Geometry check sheet. Reference: drawing and pictorial views, mm from the part's lowest x, y, z. Give positions to 0.01 mm unless a question says otherwise; leave off trailing zeros. Loops run counter-clockwise (first coordinate to the right, second up) from the corner with the lowest first, then second, coordinate; pieces in that order, holes last. Notation, with made-up numbers: M 61,-3.5 L 88,-3.5 A4 ccw 88,0.5 Z; hole C 11,74.25 d8. An arc over 180 degrees is marked long. Put each result on its own line as item: value. Start each with the question number.
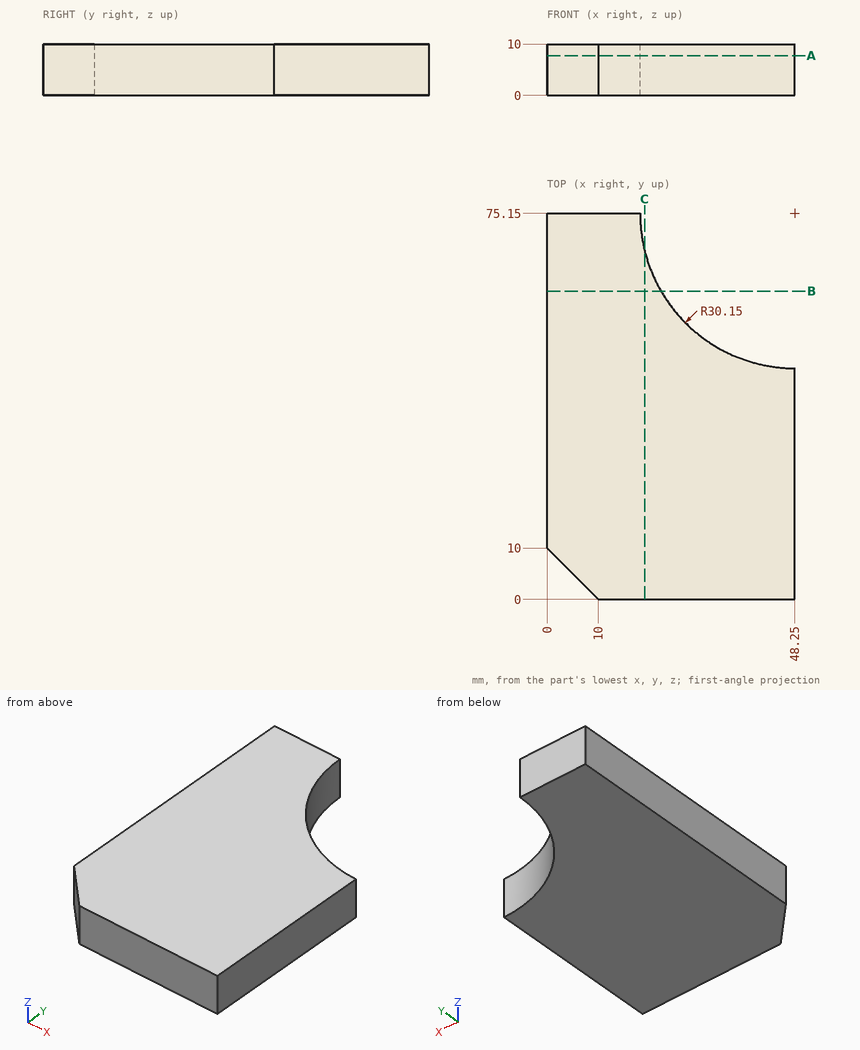
Q1. Section check A-A, the plane z = 7.75. Record the cut outline in (x, y), then the cut area to 3 significant figures.
Q2. Thickness scan on line 1 along Y through (x, z) = (29, 6); line 2 along Y through (x, z) = (37, 3.5); line 3 along X through (y, z) = (49, 3.75). Record the ranges inside material, lowest first. Write a range as [from, to].
Q3. Section check C-C, the plane x = 19. Record the cut outline in (y, z), then the cut area to 3 significant figures.
Q4. Section check B-B, the plane y = 60. Record the cut outline in (x, z), then the cut area to 3 significant figures.
Found:
1. outline: M 0,10 L 10,0 L 48.25,0 L 48.25,45 A30.15 cw 18.1,75.15 L 0,75.15 Z
1. area: 2,860 mm^2
2. line 1: y = [0, 51.95]
2. line 2: y = [0, 47.18]
2. line 3: x = [0, 33.24]
3. outline: M 0,0 L 67.84,0 L 67.84,10 L 0,10 Z
3. area: 678 mm^2
4. outline: M 0,0 L 22.18,0 L 22.18,10 L 0,10 Z
4. area: 222 mm^2
